```python
from build123d import *

# Parameters (mm, degrees)
SKETCH1_R                = 31.75
SKETCH1_W                = 44.45
SKETCH1_H                = 38.1
BASE_DEPTH               = 1.5875
TRENCH_REACH             = 11.525
SKETCH2_W                = 1.5875
SKETCH2_H                = 38.1
TRENCH_DIRECTION_2_REACH = 55.975


with BuildPart() as part:
    # Sketch1 → Base (new body, symmetric)
    with BuildSketch(Plane.XY):
        Circle(SKETCH1_R)
        Rectangle(SKETCH1_W, SKETCH1_H, mode=Mode.SUBTRACT)
    extrude(amount=BASE_DEPTH, both=True)

    # Sketch2 → Trench (cut, up to next)
    with BuildSketch(Plane.ZY.offset(-22.225), mode=Mode.PRIVATE) as trench_sk1:
        with Locations((0.79375, 0)):
            Rectangle(SKETCH2_W, SKETCH2_H)
    trench_tool1 = extrude(trench_sk1.sketch, amount=-TRENCH_REACH, mode=Mode.PRIVATE) & part.part
    add(trench_tool1.solids().sort_by_distance((22.225, 0, 0.79375))[0], mode=Mode.SUBTRACT)

    # Sketch2 → Trench direction 2 (cut, up to next)
    with BuildSketch(Plane.ZY.offset(-22.225), mode=Mode.PRIVATE) as trench_direction_2_sk1:
        with Locations((0.79375, 0)):
            Rectangle(SKETCH2_W, SKETCH2_H)
    trench_direction_2_tool1 = extrude(trench_direction_2_sk1.sketch, amount=TRENCH_DIRECTION_2_REACH, mode=Mode.PRIVATE) & part.part
    add(trench_direction_2_tool1.solids().sort_by_distance((22.225, 0, 0.79375))[0], mode=Mode.SUBTRACT)


solid = part.part
```
The listing builds one solid part. Answer for the finished solid, in the listing's coordinates (mm). A direction names the side the tool comes from. Round coordinates to 2 decimals unless told otherwise and drop trailing zeros. Order: outer loops, then holes, each group sorted by start corner. A loop starts at its lowest first (then second) coordinate and runs counter-clockwise, first axis right, second up. Notation, with made-up numbers: (-15.75, -35) - (43.25, -35) arc R28 cw to (43.25, 2) - close; hole circle Ø4 at (48, 31). An arc over 180 degrees is marked (long way). Put each result on its own line as item: value. Start each with the question number.
(1) For faces 4 (the flat face through (22.225, 0, -1)), 5 (the flat face through (0, -21, -1.588)), 6 (the flat face through (26, 0, 0)), determine the directions among +Z, -Z, +X, -X, +Y, -Y from which every point of the face is accessible in a straight line to the end or side of a thin tool.
(2) Find section C-C (z = 0.9). Give the vertices of the cut face in (x, y), plus the area to 3 significant figures.
(3) Find section A-A (x = 0). Give the vertices of the cut face in (y, z), plus the area to 3 significant figures.
(4) Given P1, Ø10.5, axis at x = -27.5, y = 5.5, coming from the +Z side; P2, Ø0.5, axis at y = -2, z = -1, coming from the +X side; P3, Ø1.6, axis at x = 12.5, z = 0.5, coming from the +Y side, each flat-ended and moving along its own axis, determine where each tip first touches the part or whether it passes through.
(5) Straight lines are drawn through the part: probe 1 along X at (y, z) = (-0.5, -1.15) (3 decimals); probe 2 along X at (y, z) = (15.5, -1.2) (3 decimals); probe 3 along Y at (x, z) = (-5.5, -0.1). For each, find the intervals that lie inside material, in ascending order. Write a range as from..to.
(6) Determine the mould class of faces 1 (the cylindrical face through (-31.72, 1.4, -0.33)), 2 (the flat face through (0, 24, 1.588)), 3 (the flat face through (0, -19.05, 0)) for opening direction Y: released by +Y, released by -Y, zero draft, split by the parting line, or undercut.
Reply:
1. face 4: +Z, -Z
1. face 5: -Z, +X, -X, +Y, -Y
1. face 6: +Z, +X, -X
2. outline: (-25.4, -19.05) arc R31.75 ccw to (25.4, -19.05) - close; (-25.4, 19.05) - (25.4, 19.05) arc R31.75 ccw to start
2. area: 902 mm^2
3. outline: (-31.75, -1.59) - (-19.05, -1.59) - (-19.05, 1.59) - (-31.75, 1.59) - close; (19.05, -1.59) - (31.75, -1.59) - (31.75, 1.59) - (19.05, 1.59) - close
3. area: 80.6 mm^2
4. P1: z = 0
4. P2: x = 31.7
4. P3: y = 29.52
5. probe 1: -31.746..-22.225, 22.225..31.746
5. probe 2: -27.709..-22.225, 22.225..27.709
5. probe 3: -31.27..-19.05, 19.05..31.27
6. face 1: split by the parting line
6. face 2: zero draft
6. face 3: undercut
